Work out the finished part from the listing and answer in its coordinate system (mm). A direction names the side the tool comes from. Round coordinates to 2 decimals unless told otherwise and drop trailing zeros. Order: outer loops, then holes, each group sorted by start corner. A loop starts at its lowest first (then second) coordinate and runs counter-clockwise, first axis right, second up. Notation, with made-up numbers: (2, 78.5) -> (53, 78.5) arc R13 cw to (53, 101.5) -> close; hole circle Ø6 at (47, 55.5). An arc over 180 degrees is marked (long way). Use a Markdown table: item, result. Add a question column.
Item 1: A cutting plane is placed at C-C, the plane x = 178. Determine the outline of the cut face in (y, z).
Item 2: Find the intervals of material crossed by L1, parallel to Y at x = 169, z = 18; L2, parallel to X at y = -53.5, z = 18.5; L3, parallel to Z at x = 178.5, y = -191, in increasing order. Write a range as [from, to].
Item 3: A cutting plane is placed at A-A, the plane z = 20. Determine the outline of the cut face in (x, y), plus the area to 3 significant figures.
Item 4: Flat-ended cylindrical pins translate along their axes: P1, Ø4, axis at y = -67.5, z = -14.5, coming from the -X side; P2, Ø1.6, axis at x = 167, y = -173.5, coming from the +Z side; P3, Ø15, axis at y = -103.5, z = -9.5, coming from the +X side; P4, Ø1.5, axis at y = -119.5, z = -17.5, coming from the -X side. Find the tip coordinate at first contact, or state that the pin passes through.
Item 5: For a pull along Y with two mould halves and no side action, classify faces 4 (the flat face through (168, -168, 7)), 5 (the flat face through (175, -340, 13)), 6 (the flat face through (175, -10, 21)) as +Y half, -Y half, draft (parallel to the pull), parting line (faces both ways), or undercut.
Item 6: A tool of negligible diameter and unlimited length cuts with its end or side. For faces 1 (the flat face through (175, -15, 16)), 2 (the flat face through (178, -168, 0)), 3 (the flat face through (183, -168, 13)), from which of +Z, -Z, +X, -X, +Y, -Y can it reach the whole face along a straight path? Write none if from no direction.
Item 7: A cutting plane is placed at B-B, the plane y = -69.5. Determine the outline of the cut face in (x, z), plus the area to 3 significant figures.
from build123d import *

# Parameters (mm, degrees)
EXTRUDE_1_DEPTH     = 26
EXTRUDE_2_DEPTH     = 19
FILLET_1_R          = 10
EXTRUDE_3_DEPTH     = 2
SKETCH_5_W          = 161
SKETCH_5_H          = 6
CUT_EXTRUDE_1_DEPTH = 52
SKETCH_6_W          = 156.446977918
SKETCH_6_H          = 480.108754565
SKETCH_6_W_2        = 20
SKETCH_6_H_2        = 20
CUT_EXTRUDE_3_DEPTH = 401
SKETCH_7_W          = 10
SKETCH_7_H          = 10
CUT_EXTRUDE_4_DEPTH = 401
EXTRUDE_5_DEPTH     = 2


with BuildPart() as part:
    # Sketch 1 → Extrude 1 (new body)
    with BuildSketch(Plane.XY):
        Polygon((-168, 0), (168, 0), (183, 0), (183, -340), (168, -340), (168, -20), (-168, -20), (-168, -340), (-183, -340), (-183, 0), align=None)
    extrude(amount=EXTRUDE_1_DEPTH)

    # Sketch 1_4 → Extrude 2 (add)
    with BuildSketch(Plane.XY):
        Polygon((172, 0), (168, 0), (168, -20), (168, -340), (172, -340), align=None)
        Polygon((-168, -20), (-168, 0), (-172, 0), (-172, -340), (-168, -340), align=None)
    extrude(amount=-EXTRUDE_2_DEPTH)

    # Fillet 1
    fillet_1_edges = [part.edges().sort_by_distance(p)[0] for p in [
        (170, 0, -19),
        (170, -340, -19),
        (-170, -340, -19),
        (-170, 0, -19),
    ]]
    fillet(fillet_1_edges, radius=FILLET_1_R)

    # Sketch 3 → Extrude 3 (add)
    with BuildSketch(Plane.ZY.offset(-168)):
        with BuildLine():
            Line((-12, -339.539392014), (-12, -0.460607986))
            ThreePointArc((-12, -0.460607986), (-13.02408013, -0.845395743), (-14, -1.339745962))
            Line((-14, -1.339745962), (-14, -338.660254038))
            ThreePointArc((-14, -338.660254038), (-13.02408013, -339.154604257), (-12, -339.539392014))
        make_face()
    extrude_3 = extrude(amount=EXTRUDE_3_DEPTH)

    # Mirror 1: Extrude 3 across plane
    add(extrude_3.mirror(Plane(origin=(0, 0, 0), x_dir=(0, 0, 1), z_dir=(1, 0, 0))))

    # Sketch 5 → Cut-Extrude 1 (cut)
    with BuildSketch(Plane(origin=(0, 0, 0), x_dir=(1, 0, 0), z_dir=(0, 1, 0))):
        with Locations((-87.5, -3)):
            Rectangle(SKETCH_5_W, SKETCH_5_H)
        with Locations((87.5, -3)):
            Rectangle(SKETCH_5_W, SKETCH_5_H)
    extrude(amount=-CUT_EXTRUDE_1_DEPTH, mode=Mode.SUBTRACT)

    # Sketch 6 → Cut-Extrude 3 (cut)
    # profile 1 of 3: a face of its own
    with BuildSketch(Plane.ZY.offset(-168)):
        with Locations((6.474112075, -134.168402936)):
            Rectangle(SKETCH_6_W, SKETCH_6_H)
        with BuildLine():
            Line((26, -20), (26, 0))
            Line((26, 0), (6, 0))
            Line((6, 0), (-9, 0))
            ThreePointArc((-9, 0), (-10.517576993, -0.115822742), (-12, -0.460607986))
            Line((-12, -0.460607986), (-12, -339.539392014))
            ThreePointArc((-12, -339.539392014), (-10.517576993, -339.884177258), (-9, -340))
            Line((-9, -340), (26, -340))
            Line((26, -340), (26, -20))
        make_face(mode=Mode.SUBTRACT)
    # profile 2 of 3: a face of its own
    with BuildSketch(Plane.ZY.offset(-168)):
        with Locations((16, -10)):
            Rectangle(SKETCH_6_W_2, SKETCH_6_H_2)
    # profile 3 of 3: a face of its own
    with BuildSketch(Plane.ZY.offset(-168)):
        with BuildLine():
            Line((26, -340), (26, -20))
            Line((26, -20), (6, -20))
            Line((6, -20), (6, 0))
            Line((6, 0), (-9, 0))
            ThreePointArc((-9, 0), (-10.517576993, -0.115822742), (-12, -0.460607986))
            Line((-12, -0.460607986), (-12, -339.539392014))
            ThreePointArc((-12, -339.539392014), (-10.517576993, -339.884177258), (-9, -340))
            Line((-9, -340), (26, -340))
        make_face()
    extrude(amount=CUT_EXTRUDE_3_DEPTH, mode=Mode.SUBTRACT)

    # Sketch 7 → Cut-Extrude 4 (cut)
    with BuildSketch(Plane.ZY.offset(-168)):
        with Locations((21, -15)):
            Rectangle(SKETCH_7_W, SKETCH_7_H)
    extrude(amount=-CUT_EXTRUDE_4_DEPTH, mode=Mode.SUBTRACT)

    # Sketch 3_3 → Extrude 5 (add)
    with BuildSketch(Plane.ZY.offset(-168)):
        with BuildLine():
            Line((-12, -339.539392014), (-12, -0.460607986))
            ThreePointArc((-12, -0.460607986), (-13.02408013, -0.845395743), (-14, -1.339745962))
            Line((-14, -1.339745962), (-14, -338.660254038))
            ThreePointArc((-14, -338.660254038), (-13.02408013, -339.154604257), (-12, -339.539392014))
        make_face()
    extrude(amount=EXTRUDE_5_DEPTH)


solid = part.part
Reported:
| question | item | result |
|---|---|---|
| 1 | outline | (-340, 0) -> (0, 0) -> (0, 26) -> (-10, 26) -> (-10, 16) -> (-20, 16) -> (-20, 26) -> (-340, 26) -> close |
| 2 | L1 | [-340, -20], [-10, 0] |
| 2 | L2 | [168, 183] |
| 2 | L3 | [0, 26] |
| 3 | outline | (168, -340) -> (183, -340) -> (183, -20) -> (168, -20) -> close; (168, -10) -> (183, -10) -> (183, 0) -> (168, 0) -> close |
| 3 | area | 4,950 mm² |
| 4 | P1 | x = 166 |
| 4 | P2 | z = -12 |
| 4 | P3 | x = 172 |
| 4 | P4 | x = 168 |
| 5 | face 4 | draft |
| 5 | face 5 | -Y half |
| 5 | face 6 | undercut |
| 6 | face 1 | +Z, +X, -X |
| 6 | face 2 | -Z, +X, +Y, -Y |
| 6 | face 3 | +Z, -Z, +X, +Y, -Y |
| 7 | outline | (166, -14) -> (168, -14) -> (168, -19) -> (172, -19) -> (172, 0) -> (183, 0) -> (183, 26) -> (168, 26) -> (168, -12) -> (166, -12) -> close |
| 7 | area | 470 mm² |
